```python
from build123d import *

# Parameters (mm, degrees)
F0_W     = 8
F0_H     = 30
F0_W_2   = 44
F0_H_2   = 8
F1_DEPTH = 224
F2_R     = 5
F3_DEPTH = 25
F4_R     = 11
F5_DEPTH = 25
F6_SIZE  = 3
F7_R     = 8
F8_R     = 8


with BuildPart() as f1:
    # F0 (on Front) → F1 (new body)
    with BuildSketch(Plane.XZ):
        with Locations((-20.8588695079, 39.1709680259)):
            Rectangle(F0_W, F0_H)
        Polygon((-16.8588695079, 24.1709680259), (-24.8588695079, 24.1709680259), (-24.8588695079, 20.1709680259), align=None)
        Polygon((27.1411304921, -20.8290319741), (-16.8588695079, 24.1709680259), (-24.8588695079, 20.1709680259), (23.1411304921, -28.8290319741), align=None)
        with Locations((49.1411304921, -24.8290319741)):
            Rectangle(F0_W_2, F0_H_2)
        Polygon((27.1411304921, -28.8290319741), (27.1411304921, -20.8290319741), (23.1411304921, -28.8290319741), align=None)
    extrude(amount=F1_DEPTH)

    # F2 (on face) → F3 (cut)
    with BuildSketch(Plane(origin=(-24.8588695079, 0, 0), x_dir=(0, -1, 0), z_dir=(-1, 0, 0))):
        with Locations((20, 44.1709680259)):
            Circle(F2_R)
        with Locations((204, 44.1709680259)):
            Circle(F2_R)
    extrude(amount=-F3_DEPTH, mode=Mode.SUBTRACT)

    # F4 (on face) → F5 (cut)
    with BuildSketch(Plane(origin=(0, 0, -28.8290319741), x_dir=(1, 0, 0), z_dir=(0, 0, -1))):
        with Locations((55.1411304921, 34)):
            Circle(F4_R)
        with Locations((55.1411304921, 190)):
            Circle(F4_R)
    extrude(amount=-F5_DEPTH, mode=Mode.SUBTRACT)

    # F6
    f6_edges = [f1.edges().sort_by_distance(p)[0] for p in [
        (-16.85887, -199, 44.170968),
        (-16.85887, -15, 44.170968),
    ]]
    chamfer(f6_edges, length=F6_SIZE)

    # F7
    f7_edges = [f1.edges().sort_by_distance(p)[0] for p in [
        (-16.85887, -112, 24.170968),
        (27.14113, -112, -20.829032),
    ]]
    fillet(f7_edges, radius=F7_R)

    # F8
    f8_edges = [f1.edges().sort_by_distance(p)[0] for p in [
        (-24.85887, -112, 20.170968),
        (23.14113, -112, -28.829032),
    ]]
    fillet(f8_edges, radius=F8_R)


solid = f1.part
```
Can you work these out from the model? Positions are in its coordinate system, mm. A direction names the side the tool comes from. Give positions to 0.01 mm unless a question says otherwise; leave off trailing zeros. Order: outer loops, then holes, each group sorted by start corner. A loop starts at its lowest first (then second) coordinate and runs counter-clockwise, first axis right, second up. Notation, with made-up numbers: M 27,39 L 76,39 A12 cw 76,60 Z; hole C 57.25,13.5 d11. An arc over 180 degrees is marked long. One line per item, written item: value.
1) I want a section at A-A, the plane y = -20. List the corners of the cut face in (x, z) for me, plus the area to 3 significant figures.
Answer sheet:
outline: M -24.86,23.44 A8 ccw -22.57,17.84 L 20.79,-26.43 A8 ccw 26.5,-28.83 L 71.14,-28.83 L 71.14,-20.83 L 30.51,-20.83 A8 cw 24.79,-18.42 L -14.58,21.84 A8 cw -16.86,27.43 L -16.86,36.17 L -19.86,39.17 L -24.86,39.17 Z; M -24.86,49.17 L -19.86,49.17 L -16.86,52.17 L -16.86,54.17 L -24.86,54.17 Z
area: 1,090 mm^2
2) I want a section at C-C, the plane x = 35.5. List the corners of the cut face in (y, z) for me.
Answer sheet:
outline: M -224,-28.83 L 0,-28.83 L 0,-20.83 L -224,-20.83 Z
3) I want a section at D-D, the plane z = 8.5. List the corners of the cut face in (x, y) for me, plus the area to 3 significant figures.
Answer sheet:
outline: M -13.43,-224 L -1.54,-224 L -1.54,0 L -13.43,0 Z
area: 2,660 mm^2
4) For P1, Ø2, axis at x = 40.5, y = -189.5, coming from the +Z side; P2, Ø8, axis at y = -154.5, z = 23.5, coming from the +X side; P3, Ø4, axis at y = -164.5, z = 6.5, coming from the -X side, each with a flat end and sliding along its axis, tell me the tip position at first contact or that it passes through.
Answer sheet:
P1: stops at z = -20.83
P2: stops at x = -12.29
P3: stops at x = -13.43
5) On a 3-axis mill with a long thin cutter (end or side, diameter ignored), from which of +Z, -Z, +X, -X, +Y, -Y can I reach the whole of each face in a straight line? I mean faces 4 (the face through (51, -110, -20.829)), 5 (the face through (-24.249, -113.568, 20.373)). Say none if no direction works.
Answer sheet:
face 4: +Z, +X, +Y, -Y
face 5: -Z, -X, +Y, -Y
6) We'd pull the mould along Y, two halves only. Please class faces 1 (the face through (-1.2, -110.43, -3.98)), 2 (the face through (53.709, -200.906, -24.885)), 3 (the face through (9, -224, -3)): released by +Y, released by -Y, zero draft, split by the parting line, or undercut.
Answer sheet:
face 1: zero draft
face 2: undercut
face 3: released by -Y
7) I want a section at B-B, the plane y = -94. List the corners of the cut face in (x, z) for me.
Answer sheet:
outline: M -24.86,23.44 A8 ccw -22.57,17.84 L 20.79,-26.43 A8 ccw 26.5,-28.83 L 71.14,-28.83 L 71.14,-20.83 L 30.51,-20.83 A8 cw 24.79,-18.42 L -14.58,21.84 A8 cw -16.86,27.43 L -16.86,54.17 L -24.86,54.17 Z
8) Please list where these lines run through material, in increasing order: line 1 along X through (y, z) = (-35, 46); line 2 along X through (y, z) = (-27, -23); line 3 along Z through (x, y) = (66.5, -131.5).
Answer sheet:
line 1: x = -24.86 to -16.86
line 2: x = 17.43 to 46.66, 63.63 to 71.14
line 3: z = -28.83 to -20.83
